Answer from the drawing. Dimensions are ordinates in mm from the lowest x, y and z of the part. Coordinates: 2 decimals unless noted, no trailing zeros. Write each loop counter-clockwise with the first axis right and the second up, starting at its lowest first coordinate (ties: lowest second). Pieces come first, ordered by that corner, then holes.
(1) The part is cut by section A-A on x = 1.75. Determine the outline of the cut face in (y, z), plus the area to 3 significant figures.
(2) For a pull along Y with two mould halves and no side action, classify the marked faces 1, 2 and 3 as +Y half, -Y half, draft (parallel to the pull), parting line (faces both ways), or undercut.
(3) The part is cut by section B-B on y = 19.5. Determine the outline of the cut face in (x, z), plus the area to 3 significant figures.
(4) The part is cut by section D-D on z = 9.5. Determine the outline of the cut face in (x, y).
(5) Straight lines are drawn through the part: line 1 (Z direction, x = 2.35, y = 11.75); line 2 (Y direction, x = 0.45, z = 10.5); line 3 (X direction, y = 3.5, z = 4.75). For each, find the intervals that lie inside material, in ascending order.
(6) Given P1, Ø1, axis at x = 2, y = 12, coming from the -Z side, flat-ended and moving along its own axis, determine where the tip first touches the part or whether it passes through.
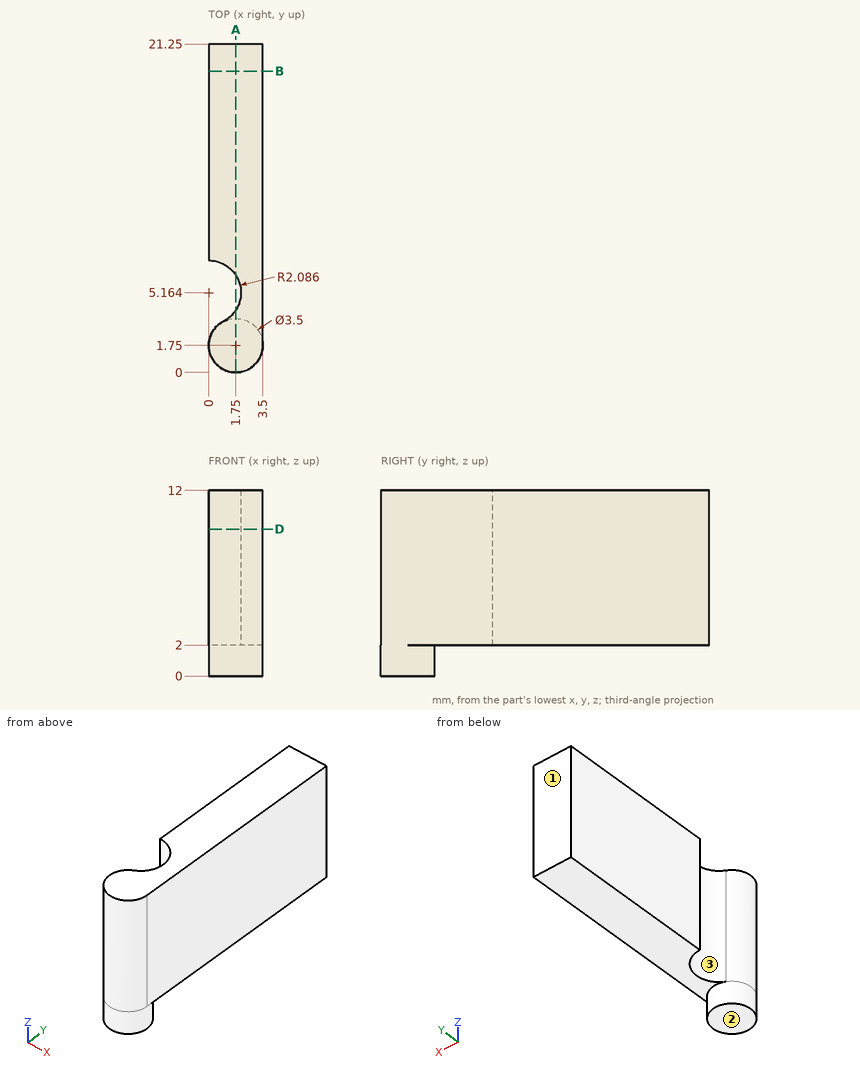
Model answer:
1. outline: (0, 0) - (3.5, 0) - (3.5, 2) - (4.03, 2) - (4.03, 12) - (0, 12) - close; (6.3, 2) - (21.25, 2) - (21.25, 12) - (6.3, 12) - close
1. area: 197 mm2
2. face 1: +Y half
2. face 2: draft
2. face 3: undercut
3. outline: (0, 2) - (3.5, 2) - (3.5, 12) - (0, 12) - close
3. area: 35.0 mm2
4. outline: (0, 7.25) arc R2.09 cw to (0.95, 3.31) arc R1.75 ccw (long way) to (3.5, 1.75) - (3.5, 21.25) - (0, 21.25) - close
5. line 1: z = 2 to 12
5. line 2: y = 0.58 to 2.92, 7.2 to 21.25
5. line 3: x = 1.26 to 3.5
6. P1: stops at z = 2
